Can you work these out from the model? Positions are in its coordinate system, mm. A direction names the side the tool comes from. Give positions to 0.01 mm unless a question says otherwise; leave off trailing zeros. Loops run counter-clockwise (first coordinate to the right, second up) from the corner with the lowest first, then second, coordinate; pieces in that order, holes last. Notation, with made-up numbers: M 38.5,37.25 L 95.5,37.25 A13 ccw 95.5,48.25 Z; hole C 36.25,-4.5 d5. An arc over 180 degrees is marked long. Put each result on its own line as item: value. Start each with the question number.
1) For P1, Ø1.2, axis at x = -1, y = 9, coming from the +Z side; P2, Ø2, axis at y = 2, z = 8.5, coming from the +X side; P3, Ø3.5, axis at x = -1.5, z = 13, coming from the +Y side, each with a flat end and sliding along its axis, tell me the tip position at first contact or that it passes through.
2) Please list where these lines run through material, in increasing order: line 1 along Y through (x, z) = (-8.5, 5.5) (3 decimals); line 2 along X through (y, z) = (-0.75, 12). Write a range as from..to.
3) If we mould it in two halves opening along X, with no side actions, what happens to faces 1 (the flat face through (6.731, 0, 18)), 2 (the flat face through (-10.795, -5, 16)), 3 (the flat face through (-9, 3.302, 18)), 4 (the flat face through (-3.302, 9, 18))? For each: +X half, -X half, draft (parallel to the pull), parting line (faces both ways), or undercut.
4) Imagine slicing it at C-C (z = 11). Write out the boundary of the cut face in (x, y) (3 decimals).
5) Imagine slicing it at A-A (x = 2.5). Write out the boundary of the cut face in (y, z) (3 decimals), then the cut area to 3 significant figures.
6) For faces 5 (the flat face through (-6.731, 0, 18)), 6 (the flat face through (3.302, -9, 18)), 7 (the flat face through (3.302, 9, 18)), which set-ups out of +Z, -Z, +X, -X, +Y, -Y let a thin tool reach every point of the face, with its end or its side?
from build123d import *

# Parameters (mm, degrees)
F1_DEPTH = 33.02
F0_W     = 4.064
F0_H     = 6.604
F0_W_2   = 6.604
F0_H_2   = 4.064
F2_DEPTH = 2.54


with BuildPart() as f1:
    # F0 (on Top) → F1 (new body)
    with BuildSketch(Plane.XY):
        Polygon((-3.302, 10.795), (-10.795, 10.795), (-10.795, 3.302), (-6.731, 3.302), (-6.731, -3.302), (-10.795, -3.302), (-10.795, -10.795), (-3.302, -10.795), (-3.302, -6.731), (3.302, -6.731), (3.302, -10.795), (10.795, -10.795), (10.795, -3.302), (6.731, -3.302), (6.731, 3.302), (10.795, 3.302), (10.795, 10.795), (3.302, 10.795), (3.302, 6.731), (-3.302, 6.731), align=None)
    extrude(amount=F1_DEPTH)

    # F0 (on Top) → F2 (join)
    with BuildSketch(Plane.XY):
        with Locations((-8.763, 0)):
            Rectangle(F0_W, F0_H)
        with Locations((0, 8.763)):
            Rectangle(F0_W_2, F0_H_2)
        with Locations((8.763, 0)):
            Rectangle(F0_W, F0_H)
        with Locations((0, -8.763)):
            Rectangle(F0_W_2, F0_H_2)
    extrude(amount=F2_DEPTH)


solid = f1.part
Recorded:
1. P1: z = 2.54
1. P2: x = 6.73
1. P3: y = 6.73
2. line 1: -10.795..-3.302, 3.302..10.795
2. line 2: -6.73..6.73
3. face 1: +X half
3. face 2: -X half
3. face 3: draft
3. face 4: undercut
4. outline: M -10.795,-10.795 L -3.302,-10.795 L -3.302,-6.731 L 3.302,-6.731 L 3.302,-10.795 L 10.795,-10.795 L 10.795,-3.302 L 6.731,-3.302 L 6.731,3.302 L 10.795,3.302 L 10.795,10.795 L 3.302,10.795 L 3.302,6.731 L -3.302,6.731 L -3.302,10.795 L -10.795,10.795 L -10.795,3.302 L -6.731,3.302 L -6.731,-3.302 L -10.795,-3.302 Z
5. outline: M -10.795,0 L 10.795,0 L 10.795,2.54 L 6.731,2.54 L 6.731,33.02 L -6.731,33.02 L -6.731,2.54 L -10.795,2.54 Z
5. area: 465 mm²
6. face 5: +Z, -X
6. face 6: +Z, -Y
6. face 7: +Z, +Y
